Geometry: see drawing. Coordinates: mm, zero at the bounding-box minimum. A direction names the side the tool comes from. Give positions to 0.01 mm unless a question says otherwise; leave off trailing zeros. Write each loop counter-clockwise with the first axis right and the second up, starting at its lowest first coordinate (ties: lowest second). Pieces come first, ordered by that corner, then holes. Notation, with made-up numbers: M 0,36.25 L 12,36.25 A33 ccw 12,72.25 Z; hole C 45.25,86.25 d2. An arc over 180 degrees is marked long. Use one line per item in the form item = value. Start each with the question number.
Item 1: Section query B-B on x = 40. Return loops of the section in (y, z).
Item 2: Access query for the marked faces 1 and 2. Directions: +Z, -Z, +X, -X, +Y, -Y. A direction counts if a zero-diameter tool reaches every point of the face in a straight line with its end or side. Return the directions, or none.
Item 3: Section query C-C on z = 26.5. Return loops of the section in (x, y).
Item 4: Section query A-A on y = 31.5. Return loops of the section in (x, z).
Item 5: Contact query for flat-ended pins moving along their axis: P1, Ø1, axis at y = 42.5, z = 13.5, coming from the -X side; P2, Ø2, axis at y = 28, z = 23.5, coming from the +X side; P3, Ø5, axis at x = 68, z = 23.5, coming from the -Y side. Output: stop coordinate, or through.
Item 6: Section query D-D on x = 62.5. Return loops of the section in (y, z).
Item 7: Material intervals for line 1 along Z through (x, y) = (40, 78); line 2 along X through (y, z) = (58, 16.5); line 3 along Y through (x, z) = (17.5, 19), sorted ascending. Write a range as from..to.
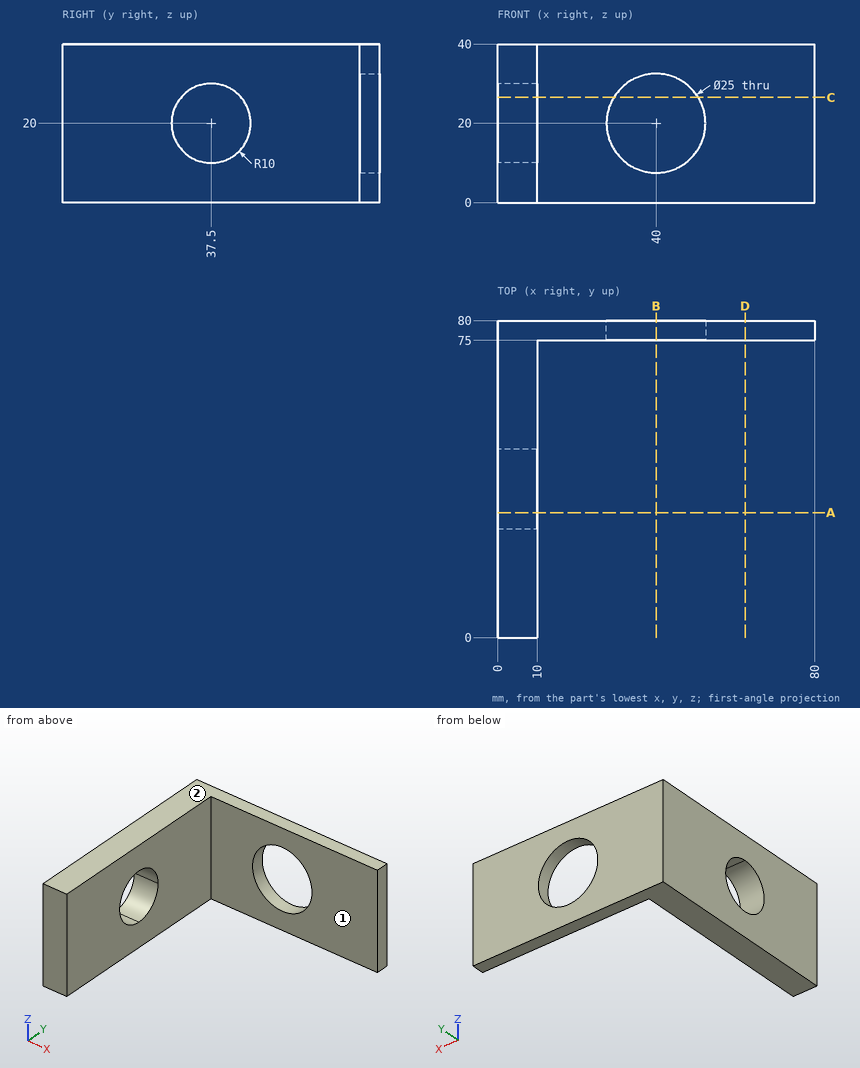
Answer sheet:
q1.outline = M 75,0 L 80,0 L 80,7.5 L 75,7.5 Z; M 75,32.5 L 80,32.5 L 80,40 L 75,40 Z
q2.face_1 = +Z, -Z, +X, -Y
q2.face_2 = +Z, +X, -X, +Y, -Y
q3.outline = M 0,0 L 10,0 L 10,29.9 L 0,29.9 Z; M 0,45.1 L 10,45.1 L 10,75 L 29.32,75 L 29.32,80 L 0,80 Z; M 50.68,75 L 80,75 L 80,80 L 50.68,80 Z
q4.outline = M 0,0 L 10,0 L 10,12 L 0,12 Z; M 0,28 L 10,28 L 10,40 L 0,40 Z
q5.P1 = through
q5.P2 = 10
q5.P3 = 75
q6.outline = M 75,0 L 80,0 L 80,40 L 75,40 Z
q7.line_1 = 0..7.5, 32.5..40
q7.line_2 = 0..10
q7.line_3 = 75..80
